```python
from build123d import *

# Parameters (mm, degrees)
F0_W     = 304.8
F0_H     = 254
F1_DEPTH = 12.7
F2_W     = 12.7
F2_H     = 304.8
F3_DEPTH = 6.35
F4_R     = 50.8
F5_W     = 50.8
F5_H     = 254
F6_DEPTH = 12.7
F7_R     = 50.79999


# Not quite as in the source:
# - a fillet or chamfer is up to 0.001 mm smaller than in the source, because OpenCascade refuses the exact size
# - a feature of the source that left no trace in its solid (it failed there, or was rolled back) is left out


with BuildPart() as f1:
    # F0 (on Top) → F1 (new body)
    with BuildSketch(Plane.XY):
        Polygon((304.8, 127), (304.8, 152.4), (-304.8, 152.4), (-304.8, -152.4), (304.8, -152.4), (304.8, -127), (203.2, -127), (203.2, 127), align=None)
        Rectangle(F0_W, F0_H, mode=Mode.SUBTRACT)
    extrude(amount=F1_DEPTH)

    # F2 (on face) → F3 (cut)
    with BuildSketch(Plane.XY.offset(12.7)):
        with Locations((-228.6, 0)):
            Rectangle(F2_W, F2_H)
    extrude(amount=-F3_DEPTH, mode=Mode.SUBTRACT)

    # F4
    f4_edges = [f1.edges().sort_by_distance(p)[0] for p in [
        (203.2, -127, 6.35),
        (203.2, 127, 6.35),
    ]]
    fillet(f4_edges, radius=F4_R)

    # F5 (on face) → F6 (cut)
    with BuildSketch(Plane.XY.offset(12.7)):
        with Locations((-279.4, 0)):
            Rectangle(F5_W, F5_H)
    extrude(amount=-F6_DEPTH, mode=Mode.SUBTRACT)

    # F7 (radius 50.8 in the source; OpenCascade refuses exactly that, so slightly less here)
    f7_edges = [f1.edges().sort_by_distance(p)[0] for p in [
        (-254, 127, 6.35),
        (-254, -127, 6.35),
    ]]
    fillet(f7_edges, radius=F7_R)


solid = f1.part
```
For this review, take the finished solid that the model builds, in its own axes (mm). A direction names the side the tool comes from. Round coordinates to 2 decimals unless told otherwise and drop trailing zeros. Write each loop counter-clockwise with the first axis right and the second up, starting at its lowest first coordinate (ties: lowest second). Pieces come first, ordered by that corner, then holes. Notation, with made-up numbers: (22, 85) -> (70, 85) arc R16 cw to (70, 97) -> close; hole circle Ø8 at (82.5, 5.25). An arc over 180 degrees is marked (long way). Use one line per item in the form item = value.
1) Take a section at A-A, the plane z = 10.5. Count the separate pieces of the cut face and the enclosed holes in it, and give its area (3 significant figures).
Found:
separate_pieces = 2
enclosed_holes = 1
area = 68,000 mm2
2) Take a section at C-C, the plane y = -52.5. Write out the cut boundary in (x, z).
Found:
outline = (-254, 0) -> (-152.4, 0) -> (-152.4, 12.7) -> (-222.25, 12.7) -> (-222.25, 6.35) -> (-234.95, 6.35) -> (-234.95, 12.7) -> (-254, 12.7) -> close; (152.4, 0) -> (203.2, 0) -> (203.2, 12.7) -> (152.4, 12.7) -> close
3) Take a section at D-D, the plane y = 96.5. Write out the cut boundary in (x, z).
Found:
outline = (-258.23, 0) -> (-152.4, 0) -> (-152.4, 12.7) -> (-222.25, 12.7) -> (-222.25, 6.35) -> (-234.95, 6.35) -> (-234.95, 12.7) -> (-258.23, 12.7) -> close; (152.4, 0) -> (207.43, 0) -> (207.43, 12.7) -> (152.4, 12.7) -> close
4) Mouldability with a two-part tool opening along X and no side actions: class faces 1 (the cylindrical face through (217.686, -111.724, 6.439)), 2 (the flat face through (-4, -152.4, 6)), 3 (the flat face through (-2, -127, 6)) as +X half, -X half, draft (parallel to the pull), parting line (faces both ways), or undercut.
Found:
face_1 = +X half
face_2 = draft
face_3 = undercut
5) Clearance check with flat-ended pins moving along their axes: pin 1 (5 mm diameter, centred on y = 40.5, z = 8, fed in from -X); pin 2 (6.5 mm diameter, centred on y = -20.5, z = 4.5, fed in from +X); pin 3 (6.5 mm diameter, centred on x = -227, y = 28, fed in from +Z). State where each tip first meets the part, or that it passes through.
Found:
pin_1 = -254
pin_2 = 203.2
pin_3 = 6.35
6) Take a section at B-B, the plane x = 98. Write out the cut boundary in (y, z), and give its area (3 significant figures).
Found:
outline = (-152.4, 0) -> (-127, 0) -> (-127, 12.7) -> (-152.4, 12.7) -> close; (127, 0) -> (152.4, 0) -> (152.4, 12.7) -> (127, 12.7) -> close
area = 645 mm2
7) To check wall thickness, follow L1, parallel to X at y = -79.5, z = 9; L2, parallel to Y at x = -120, z = 11.5; L3, parallel to X at y = -9, z = 11.5. State the ranges of each line that lie inside material, in increasing order. Write a range as from..to.
Found:
L1 = -254.11..-234.95, -222.25..-152.4, 152.4..203.31
L2 = -152.4..-127, 127..152.4
L3 = -254..-234.95, -222.25..-152.4, 152.4..203.2
8) Tool access review of faces 4 (the cylindrical face through (218.476, 112.514, 6.439)), 5 (the flat face through (-229, 2, 6.35)), 6 (the flat face through (152.4, -2, 6)): name each direction out of +Z, -Z, +X, -X, +Y, -Y from which nothing blocks a thin tool from reaching the whole face with its end or side.
Found:
face_4 = +Z, -Z, +X
face_5 = +Z, +Y, -Y
face_6 = +Z, -Z
